The model under review builds one solid part; all positions refer to its coordinate system, in mm. Coordinates: 2 decimals unless noted, no trailing zeros. Order: outer loops, then holes, each group sorted by start corner. A loop starts at its lowest first (then second) coordinate and runs counter-clockwise, first axis right, second up. Notation, with made-up numbers: (78, -20.5) - (108, -20.5) arc R17 ccw to (108, -0.5) - close; hole circle Ø5 at (5.5, -25). An arc over 180 degrees is marked (long way). Answer in a Markdown table with one row per item.
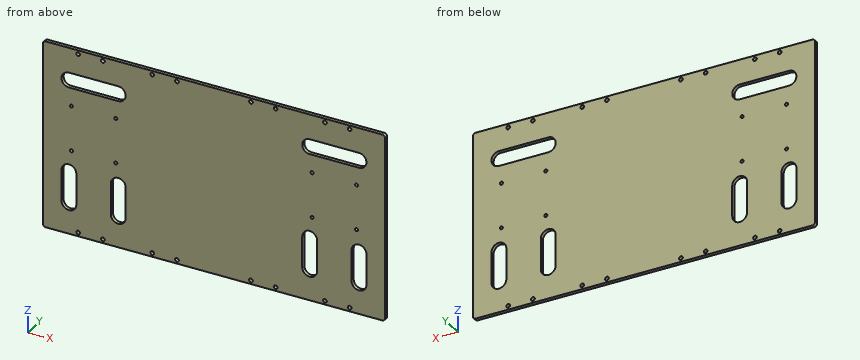
```python
from build123d import *

# Parameters (mm, degrees)
SKETCH_1_W             = 277.163859754
SKETCH_1_H             = 150
EXTRUDE_1_DEPTH        = 3
SKETCH_2_R             = 1.5
CUT_EXTRUDE_1_DEPTH    = 10
CUT_EXTRUDE_2_DEPTH    = 10
FILLET_1_R             = 2
SKETCH_4_R             = 1.25
CUT_EXTRUDE_2556_DEPTH = 10


with BuildPart() as part:
    # 草图1 → 凸台-拉伸1 (new body)
    with BuildSketch(Plane(origin=(0, 0, 0), x_dir=(1, 0, 0), z_dir=(0, 1, 0))):
        with Locations((0, 132.402514855)):
            Rectangle(SKETCH_1_W, SKETCH_1_H)
    extrude(amount=EXTRUDE_1_DEPTH)

    # 草图2 → 切除-拉伸1 (cut)
    with BuildSketch(Plane(origin=(0, 3, 0), x_dir=(1, 0, 0), z_dir=(0, 1, 0))):
        with Locations(Location((-50, 60.402514855, 0), (0, 0, 270))):
            Circle(SKETCH_2_R)
        with Locations(Location((-30, 60.402514855, 0), (0, 0, 270))):
            Circle(SKETCH_2_R)
        with Locations(Location((-110, 60.402514855, 0), (0, 0, 270))):
            Circle(SKETCH_2_R)
        with Locations(Location((-90, 60.402514855, 0), (0, 0, 270))):
            Circle(SKETCH_2_R)
        with Locations(Location((90, 60.402514855, 0), (0, 0, 90))):
            Circle(SKETCH_2_R)
        with Locations(Location((110, 60.402514855, 0), (0, 0, 90))):
            Circle(SKETCH_2_R)
        with Locations(Location((30, 60.402514855, 0), (0, 0, 90))):
            Circle(SKETCH_2_R)
        with Locations(Location((50, 60.402514855, 0), (0, 0, 90))):
            Circle(SKETCH_2_R)
        with Locations(Location((50, 204.402514855, 0), (0, 0, 270))):
            Circle(SKETCH_2_R)
        with Locations(Location((30, 204.402514855, 0), (0, 0, 270))):
            Circle(SKETCH_2_R)
        with Locations(Location((110, 204.402514855, 0), (0, 0, 270))):
            Circle(SKETCH_2_R)
        with Locations(Location((90, 204.402514855, 0), (0, 0, 270))):
            Circle(SKETCH_2_R)
        with Locations(Location((-90, 204.402514855, 0), (0, 0, 90))):
            Circle(SKETCH_2_R)
        with Locations(Location((-110, 204.402514855, 0), (0, 0, 90))):
            Circle(SKETCH_2_R)
        with Locations(Location((-30, 204.402514855, 0), (0, 0, 90))):
            Circle(SKETCH_2_R)
        with Locations(Location((-50, 204.402514855, 0), (0, 0, 90))):
            Circle(SKETCH_2_R)
    extrude(amount=-CUT_EXTRUDE_1_DEPTH, mode=Mode.SUBTRACT)

    # 草图3 → 切除-拉伸2 (cut)
    with BuildSketch(Plane(origin=(0, 3, 0), x_dir=(1, 0, 0), z_dir=(0, 1, 0))):
        with BuildLine():
            Line((-117.581929877, 89.402514855), (-77.581929877, 89.402514855))
            ThreePointArc((-77.581929877, 89.402514855), (-71.581929877, 83.402514855), (-77.581929877, 77.402514855))
            Line((-77.581929877, 77.402514855), (-117.581929877, 77.402514855))
            ThreePointArc((-117.581929877, 77.402514855), (-123.581929877, 83.402514855), (-117.581929877, 89.402514855))
        make_face()
        with BuildLine():
            Line((-111.581929877, 182.402514855), (-111.581929877, 157.402514855))
            ThreePointArc((-111.581929877, 157.402514855), (-117.581929877, 151.402514855), (-123.581929877, 157.402514855))
            Line((-123.581929877, 157.402514855), (-123.581929877, 182.402514855))
            ThreePointArc((-123.581929877, 182.402514855), (-117.581929877, 188.402514855), (-111.581929877, 182.402514855))
        make_face()
        with BuildLine():
            Line((-71.581929877, 182.402514855), (-71.581929877, 157.402514855))
            ThreePointArc((-71.581929877, 157.402514855), (-77.581929877, 151.402514855), (-83.581929877, 157.402514855))
            Line((-83.581929877, 157.402514855), (-83.581929877, 182.402514855))
            ThreePointArc((-83.581929877, 182.402514855), (-77.581929877, 188.402514855), (-71.581929877, 182.402514855))
        make_face()
        with BuildLine():
            Line((117.581929877, 89.402514855), (77.581929877, 89.402514855))
            ThreePointArc((77.581929877, 89.402514855), (71.581929877, 83.402514855), (77.581929877, 77.402514855))
            Line((77.581929877, 77.402514855), (117.581929877, 77.402514855))
            ThreePointArc((117.581929877, 77.402514855), (123.581929877, 83.402514855), (117.581929877, 89.402514855))
        make_face()
        with BuildLine():
            Line((111.581929877, 182.402514855), (111.581929877, 157.402514855))
            ThreePointArc((111.581929877, 157.402514855), (117.581929877, 151.402514855), (123.581929877, 157.402514855))
            Line((123.581929877, 157.402514855), (123.581929877, 182.402514855))
            ThreePointArc((123.581929877, 182.402514855), (117.581929877, 188.402514855), (111.581929877, 182.402514855))
        make_face()
        with BuildLine():
            Line((71.581929877, 182.402514855), (71.581929877, 157.402514855))
            ThreePointArc((71.581929877, 157.402514855), (77.581929877, 151.402514855), (83.581929877, 157.402514855))
            Line((83.581929877, 157.402514855), (83.581929877, 182.402514855))
            ThreePointArc((83.581929877, 182.402514855), (77.581929877, 188.402514855), (71.581929877, 182.402514855))
        make_face()
    extrude(amount=-CUT_EXTRUDE_2_DEPTH, mode=Mode.SUBTRACT)

    # 圆角1
    fillet_1_edges = [part.edges().sort_by_distance(p)[0] for p in [
        (-138.581929877, 1.5, -207.402514855),
        (138.581929877, 1.5, -207.402514855),
        (138.581929877, 1.5, -57.402514855),
        (-138.581929877, 1.5, -57.402514855),
    ]]
    fillet(fillet_1_edges, radius=FILLET_1_R)

    # 草图4 → Cut-Extrude 2556 (cut)
    with BuildSketch(Plane(origin=(0, 3, 0), x_dir=(1, 0, 0), z_dir=(0, 1, 0))):
        with Locations(Location((-115.581929877, 139.902514855, 0), (0, 0, 270))):
            Circle(SKETCH_4_R)
        with Locations(Location((-79.581929877, 139.902514855, 0), (0, 0, 270))):
            Circle(SKETCH_4_R)
        with Locations(Location((-79.581929877, 103.902514855, 0), (0, 0, 270))):
            Circle(SKETCH_4_R)
        with Locations(Location((-115.581929877, 103.902514855, 0), (0, 0, 270))):
            Circle(SKETCH_4_R)
        with Locations(Location((115.581929877, 103.902514855, 0), (0, 0, 90))):
            Circle(SKETCH_4_R)
        with Locations(Location((79.581929877, 103.902514855, 0), (0, 0, 90))):
            Circle(SKETCH_4_R)
        with Locations(Location((79.581929877, 139.902514855, 0), (0, 0, 90))):
            Circle(SKETCH_4_R)
        with Locations(Location((115.581929877, 139.902514855, 0), (0, 0, 90))):
            Circle(SKETCH_4_R)
    extrude(amount=-CUT_EXTRUDE_2556_DEPTH, mode=Mode.SUBTRACT)


solid = part.part
```
Item 1: We need section B-B, the plane z = -85.5. Write out the cut boundary in (x, y).
Check values:
| item | result |
|---|---|
| outline | (-138.58, 0) - (-123.2, 0) - (-123.2, 3) - (-138.58, 3) - close; (-71.96, 0) - (71.96, 0) - (71.96, 3) - (-71.96, 3) - close; (123.2, 0) - (138.58, 0) - (138.58, 3) - (123.2, 3) - close |
Item 2: We need section A-A, the plane x = 103. Write out the cut boundary in (y, z).
Check values:
| item | result |
|---|---|
| outline | (0, -207.4) - (3, -207.4) - (3, -89.4) - (0, -89.4) - close; (0, -77.4) - (3, -77.4) - (3, -57.4) - (0, -57.4) - close |
Item 3: We need section C-C, the plane y = 1.1. State how many separate pieces and enclosed holes the cut face has, then the cut area to 3 significant figures.
Check values:
| item | result |
|---|---|
| separate pieces | 1 |
| enclosed holes | 30 |
| area | 38,600 mm^2 |
Item 4: To check wall thickness, follow line 1 (X direction, y = 1.3, z = -159.5); line 2 (Z direction, x = -110, y = 1.7); line 3 (Z direction, x = 103.5, y = 0.6). State the ranges of each line that lie inside material, in increasing order. Write a range as from..to.
Check values:
| item | result |
|---|---|
| line 1 | -138.58..-123.58, -111.58..-83.58, -71.58..71.58, 83.58..111.58, 123.58..138.58 |
| line 2 | -207.4..-205.9, -202.9..-89.4, -77.4..-61.9, -58.9..-57.4 |
| line 3 | -207.4..-89.4, -77.4..-57.4 |
